```python
from build123d import *

# Parameters (mm, degrees)
SKETCH1_W                = 110
SKETCH1_H                = 18
BOSS_EXTRUDE1_DEPTH      = 9
SKETCH2_W                = 41
SKETCH2_H                = 2
CUT_EXTRUDE1_DEPTH       = 112.825757319
F_8_0_8_DIAMETER_HOLE1_D = 8
M8_TAPPED_HOLE1_D        = 6.8
CHAMFER1_SIZE            = 1


with BuildPart() as part:
    # Sketch1 → Boss-Extrude1 (new, symmetric)
    with BuildSketch(Plane.XY):
        with Locations((55, 0)):
            Rectangle(SKETCH1_W, SKETCH1_H)
    extrude(amount=BOSS_EXTRUDE1_DEPTH, both=True)

    # Sketch2 → Cut-Extrude1 (cut, through all)
    with BuildSketch(Plane.XY.offset(9)):
        with Locations((89.5, 8)):
            Rectangle(SKETCH2_W, SKETCH2_H)
    extrude(amount=-CUT_EXTRUDE1_DEPTH, mode=Mode.SUBTRACT)

    # Ø8.0 (8) Diameter Hole1 (through all)
    with Locations(Plane.XY.offset(9)):
        with Locations((33, 0)):
            Hole(F_8_0_8_DIAMETER_HOLE1_D / 2)

    # M8 Tapped Hole1 (through all)
    with Locations(Plane(origin=(0, 9, 0), x_dir=(1, 0, 0), z_dir=(0, 1, 0))):
        with Locations((21, 0), (57, 0), (80, 0), (100, 0)):
            Hole(M8_TAPPED_HOLE1_D / 2)

    # Chamfer1
    chamfer1_edges = [part.edges().sort_by_distance(p)[0] for p in [
        (110, -1, 9),
        (110, 7, 0),
        (0, 0, 9),
        (110, -1, -9),
        (0, 0, -9),
        (0, 9, 0),
        (110, -9, 0),
        (0, -9, 0),
    ]]
    chamfer(chamfer1_edges, length=CHAMFER1_SIZE)


solid = part.part
```
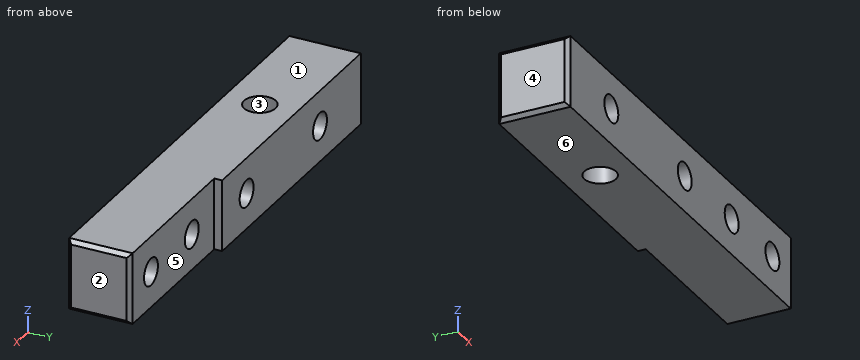
Here's how the part is built. I have some questions about the finished solid (model axes, mm). Face numbers are marked on the shaded views. A direction names the side the tool comes from. Coordinates: 2 decimals unless noted, no trailing zeros. Order: outer loops, then holes, each group sorted by start corner. A loop starts at its lowest first (then second) coordinate and runs counter-clockwise, first axis right, second up. Notation, with made-up numbers: (7, 73.5) -> (14, 73.5) arc R18 cw to (14, 100.5) -> close; hole circle Ø10 at (-8.5, -27.5). An arc over 180 degrees is marked (long way). Return JSON: item names as keys, results as strings.
1) If we section it at A-A on z = 0: List the corners of the cut face in (x, y) for me.
Conclusion:
{"outline": "(0, -8) -> (1, -9) -> (17.6, -9) -> (17.6, 9) -> (1, 9) -> (0, 8) -> close; (24.4, -9) -> (53.6, -9) -> (53.6, 9) -> (24.4, 9) -> close; (60.4, -9) -> (76.6, -9) -> (76.6, 7) -> (69, 7) -> (69, 9) -> (60.4, 9) -> close; (83.4, -9) -> (96.6, -9) -> (96.6, 7) -> (83.4, 7) -> close; (103.4, -9) -> (109, -9) -> (110, -8) -> (110, 6) -> (109, 7) -> (103.4, 7) -> close; hole circle Ø8 at (33, 0)"}
2) If I drill on probe 1 along Z at (x, y) = (57, -3); probe 2 along Y at (x, z) = (33, 2.5); probe 3 along Y at (x, z) = (97, 4), over which ranges is the centre line in solid material (lowest first)?
Conclusion:
{"probe 1": "z = -9 to -3.4, 3.4 to 9", "probe 2": "y = -9 to -4, 4 to 9", "probe 3": "y = -9 to 7"}
3) If we section it at B-B on x = 80: List the corners of the cut face in (y, z) for me.
Conclusion:
{"outline": "(-9, -9) -> (7, -9) -> (7, -3.4) -> (-9, -3.4) -> close; (-9, 3.4) -> (7, 3.4) -> (7, 9) -> (-9, 9) -> close"}
4) Thinking about a two-plate mould opening in X: for the marked faces 1, 2, 3 and 4, which applies, +X half, -X half, draft (parallel to the pull), parting line (faces both ways), or undercut?
Conclusion:
{"face 1": "draft", "face 2": "+X half", "face 3": "undercut", "face 4": "-X half"}
5) If we section it at D-D on y = -5.5: List the corners of the cut face in (x, z) for me.
Conclusion:
{"outline": "(0, -8) -> (1, -9) -> (109, -9) -> (110, -8) -> (110, 8) -> (109, 9) -> (1, 9) -> (0, 8) -> close; hole circle Ø6.8 at (21, 0); hole circle Ø6.8 at (57, 0); hole circle Ø6.8 at (80, 0); hole circle Ø6.8 at (100, 0)"}
6) I'm going to push flat-ended pins straight in: P1, Ø8, axis at x = 100, z = 0, coming from the -Y side; P2, Ø5.5, axis at x = 80.5, z = -3, coming from the +Y side. Where does each tip first touch, or does it pass through?
Conclusion:
{"P1": "stops at y = -9", "P2": "stops at y = 7"}
7) If we section it at C-C on y = 0: List the corners of the cut face in (x, z) for me.
Conclusion:
{"outline": "(0, -8) -> (1, -9) -> (29, -9) -> (29, 9) -> (1, 9) -> (0, 8) -> close; (37, -9) -> (109, -9) -> (110, -8) -> (110, 8) -> (109, 9) -> (37, 9) -> close; hole circle Ø6.8 at (21, 0); hole circle Ø6.8 at (57, 0); hole circle Ø6.8 at (80, 0); hole circle Ø6.8 at (100, 0)"}
8) On a 3-axis mill with a long thin cutter (end or side, diameter ignored), from which of +Z, -Z, +X, -X, +Y, -Y can I reach the whole of each face in a straight line? I mean the marked faces 5 and 6. Say none if no direction works.
Conclusion:
{"face 5": "+Z, -Z, +X, +Y", "face 6": "-Z, +X, -X, +Y, -Y"}
